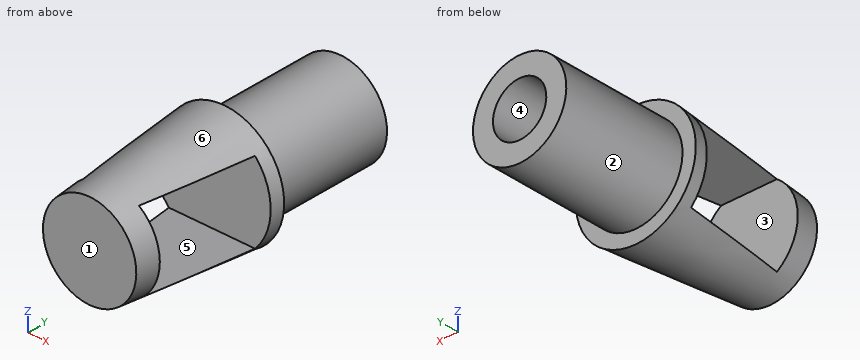
```python
from build123d import *

# Parameters (mm, degrees)
SKETCH1_W               = 3
SKETCH1_H               = 19
SKETCH2_W               = 12
SKETCH2_H               = 16.5
CUT_EXTRUDE1_DEPTH      = 10
CUT_EXTRUDE1_DEPTH_BACK = 10


with BuildPart() as part:
    # Sketch1 → Revolve1 (revolve)
    with BuildSketch(Plane(origin=(0, 0, 0), x_dir=(0, 0, -1), z_dir=(1, 0, 0))):
        with Locations((5.5, 9.5)):
            Rectangle(SKETCH1_W, SKETCH1_H)
        Polygon((7, 0), (4, 0), (0, 0), (0, -22), (7, -22), (9, 0), align=None)
    revolve(axis=Axis((0, 13.924528302, 0), (0, -1, 0)))

    # Sketch2 → Cut-Extrude1 (cut, two sides)
    with BuildSketch(Plane(origin=(0, 0, 0), x_dir=(0, 0, -1), z_dir=(1, 0, 0))) as cut_extrude1_sk:
        with Locations((0, -10.25)):
            Rectangle(SKETCH2_W, SKETCH2_H)
    extrude(amount=CUT_EXTRUDE1_DEPTH, mode=Mode.SUBTRACT)
    extrude(cut_extrude1_sk.sketch, amount=-CUT_EXTRUDE1_DEPTH_BACK, mode=Mode.SUBTRACT)


solid = part.part
```
Could you check a few things on this model? Use its own coordinates, in mm. Face numbers are marked on the shaded views. A direction names the side the tool comes from. Round coordinates to 2 decimals unless told otherwise and drop trailing zeros. Write each loop counter-clockwise with the first axis right and the second up, starting at its lowest first coordinate (ties: lowest second). Pieces come first, ordered by that corner, then holes. Notation, with made-up numbers: M 77.5,52 L 86.5,52 A24 cw 86.5,69 Z; hole C 53,-25 d7. An arc over 180 degrees is marked long. Answer in a Markdown table with one row per item. Add a question column.
Q1. Imagine slicing it at C-C (y = 4). Please give me the cut outline in (x, z).
Q2. Will these pins go through, and if not, where does the flat tip stop? pin 1 Ø8 at (y, z) = (-3.5, 4.5) entering from -X; pin 2 Ø4 at (x, y) = (2, -9) entering from -Z; pin 3 Ø6.5 at (x, y) = (-1, -7) entering from -Z.
Q3. If we mould it in two halves opening along X, with no side actions, what happens to the marked faces 4, 5 and 6? For each: +X half, -X half, draft (parallel to the pull), parting line (faces both ways), or undercut.
Q4. Imagine slicing it at D-D (y = -9). Please give me the cut outline in (x, z), then the cut area to 3 significant figures.
Q5. On a 3-axis mill with a long thin cutter (end or side, diameter ignored), from which of +Z, -Z, +X, -X, +Y, -Y can I reach the whole of each face in a straight line? I mean the marked faces 1, 2 and 3. Say none if no direction works.
Q6. Imagine slicing it at A-A (x = 0). Please give me the cut outline in (y, z).
Q7. Imagine slicing it at B-B (z = 0). Please give me the cut outline in (x, y), then the cut area to 3 significant figures.
Q8. If I drill on line 1 (X direction, y = 11, z = 0); line 2 (Y direction, x = -4.5, z = -1.25); line 3 (Y direction, x = -1, z = 1.25), over which ranges is the centre line in solid material (lowest first)? Write a range as from..to.
Values:
| question | item | result |
|---|---|---|
| 1 | outline | C 0,0 d14; hole C 0,0 d8 |
| 2 | pin 1 | x = -8.81 |
| 2 | pin 2 | z = -8.29 |
| 2 | pin 3 | z = -8.65 |
| 3 | face 4 | undercut |
| 3 | face 5 | draft |
| 3 | face 6 | parting line |
| 4 | outline | M -5.56,-6 A8.18 ccw 5.56,-6 Z; M -5.56,6 L 5.56,6 A8.18 ccw Z |
| 4 | area | 33.3 mm^2 |
| 5 | face 1 | +Z, -Z, +X, -X, -Y |
| 5 | face 2 | +Y |
| 5 | face 3 | +X, -X |
| 6 | outline | M -22,-7 L 0,-9 L 0,-7 L 19,-7 L 19,-4 L 0,-4 L 0,4 L 19,4 L 19,7 L 0,7 L 0,9 L -22,7 Z; hole M -18.5,-6 L -2,-6 L -2,6 L -18.5,6 Z |
| 7 | outline | M -9,0 L -8.82,-2 L 8.82,-2 L 9,0 L 7,0 L 7,19 L 4,19 L 4,0 L -4,0 L -4,19 L -7,19 L -7,0 Z; M -7.32,-18.5 L -7,-22 L 7,-22 L 7.32,-18.5 Z |
| 7 | area | 200 mm^2 |
| 8 | line 1 | -7..-4, 4..7 |
| 8 | line 2 | -22..-18.5, -2..19 |
| 8 | line 3 | -22..-18.5, -2..0 |
